Could you check a few things on this drawing? It's one solid part, dimensions in mm from its lowest x, y, z. Coordinates: 2 decimals unless noted, no trailing zeros. Order: outer loops, then holes, each group sorted by start corner. A loop starts at its lowest first (then second) coordinate and runs counter-clockwise, first axis right, second up. Notation, with made-up numbers: (66, -14.5) - (117, -14.5) arc R19 cw to (117, 3.5) - close; hole circle Ø3 at (65, 67.25). An arc over 180 degrees is marked (long way). Answer in a Markdown table with one row per item. Add a question column.
Item 1: Thinking about a two-plate mould opening in X: for the marked faces 1, 2 and 3, which applies, +X half, -X half, draft (parallel to the pull), parting line (faces both ways), or undercut?
Item 2: I want a section at D-D (z = 9). Please give me the cut outline in (x, y).
Item 3: Will these pins go through, and if not, where does the flat tip stop? pin 1 Ø8 at (x, y) = (10, 108) entering from -Z; pin 2 Ø8 at (y, z) = (90, 33) entering from -X; pin 3 Ø1 at (y, z) = (41, 23.5) entering from -X.
Item 4: I want a section at C-C (y = 21). Please give me the cut outline in (x, z) (3 decimals).
Item 5: If I drill on line 1 along Y through (x, z) = (39, 33); line 2 along X through (y, z) = (112, 38); line 3 along X through (y, z) = (88.5, 34), over which ranges is the centre line in solid material (lowest first)? Write a range as from..to.
Item 6: I want a section at A-A (x = 35.5). Please give me the cut outline in (y, z), plus the area to 3 significant figures.
Item 7: I want a section at B-B (z = 70.5). Please give me the cut outline in (x, y) (3 decimals), plus the area to 3 significant figures.
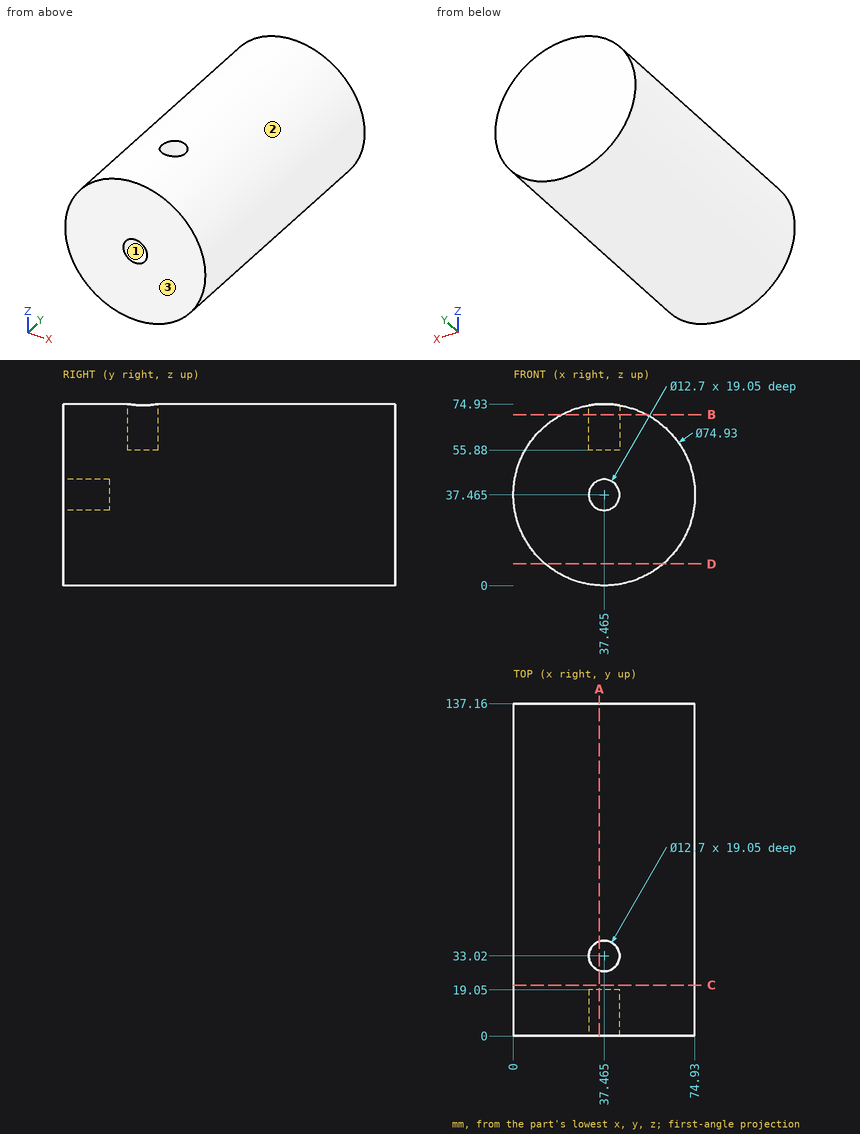
Values follow:
| question | item | result |
|---|---|---|
| 1 | face 1 | undercut |
| 1 | face 2 | parting line |
| 1 | face 3 | draft |
| 2 | outline | (13.11, 0) - (61.82, 0) - (61.82, 137.16) - (13.11, 137.16) - close |
| 3 | pin 1 | stops at z = 8.26 |
| 3 | pin 2 | stops at x = 0 |
| 3 | pin 3 | stops at x = 2.5 |
| 4 | outline | circle Ø74.93 at (37.465, 37.465) |
| 5 | line 1 | y = 19.05..137.16 |
| 5 | line 2 | x = 0..74.93 |
| 5 | line 3 | x = 0.16..74.77 |
| 6 | outline | (0, 0.05) - (137.16, 0.05) - (137.16, 74.88) - (39.06, 74.88) - (39.06, 55.88) - (26.98, 55.88) - (26.98, 74.88) - (0, 74.88) - (0, 43.5) - (19.05, 43.5) - (19.05, 31.43) - (0, 31.43) - close |
| 6 | area | 9,800 mm^2 |
| 7 | outline | (19.793, 0) - (55.137, 0) - (55.137, 137.16) - (19.793, 137.16) - close; hole circle Ø12.7 at (37.465, 33.02) |
| 7 | area | 4,720 mm^2 |
